The listing builds one solid part. Answer for the finished solid, in the listing's coordinates (mm). Face numbers are marked on the shaded views. A direction names the side the tool comes from. Coordinates: 2 decimals unless noted, no trailing zeros. Order: outer loops, then holes, each group sorted by start corner. A loop starts at its lowest first (then second) coordinate and runs counter-clockwise, first axis right, second up. Notation, with made-up numbers: (6, 40.25) - (36, 40.25) arc R18 ccw to (36, 47.25) - close; hole circle Ø6 at (48.25, 89). An arc over 180 degrees is marked (long way). Use a Markdown table: item, result. Add a question column.
Item 1: The part is cut by section C-C, the plane y = -17. Give the vertices of the cut face in (x, z).
Item 2: The part is cut by section B-B, the plane z = 0. Give the vertices of the cut face in (x, y).
Item 3: For the marked faces 4, 5, 6 and 7, determine the directions among +Z, -Z, +X, -X, +Y, -Y from which every point of the face is accessible in a straight line to the end or side of a thin tool.
Item 4: The part is cut by section D-D, the plane z = 48. Give the vertices of the cut face in (x, y), then the cut area to 3 significant figures.
Item 5: The part is cut by section A-A, the plane x = 0. Give the vertices of the cut face in (y, z).
Item 6: Find the intervals of material crossed by line 1 along Z through (x, y) = (0, -13); line 2 along Z through (x, y) = (5, -23.25); line 3 along X through (y, z) = (-10.25, -48), in increasing order.
Item 7: The mould has two halves that part along X. Classify the marked faces 1, 2 and 3: released by +X, released by -X, zero draft, split by the parting line, or undercut.
Item 8: Flat-ended cylindrical pins translate along their axes: P1, Ø4, axis at y = -14, z = 22.5, coming from the -X side; P2, Ø5.5, axis at y = -6.5, z = 55.5, coming from the -X side; P3, Ø15, axis at x = -50, y = -12, coming from the +Z side; P4, Ø23, axis at x = 0, z = 0, coming from the -Y side. Find the tip coordinate at first contact, or state that the pin passes through.
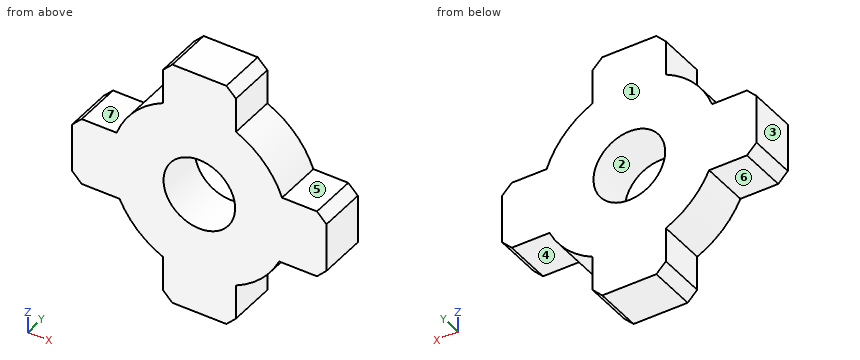
from build123d import *

# Parameters (mm, degrees)
F1_DEPTH = 25.4
F3_D     = 38.1
F4_SIZE  = 5.08
F5_SIZE  = 5.08
F6_SIZE  = 5.08
F7_SIZE  = 5.08
F8_SIZE  = 5.08
F9_SIZE  = 5.08
F10_SIZE = 5.08
F11_SIZE = 5.08


with BuildPart() as f1:
    # F0 (on Front) → F1 (new body)
    with BuildSketch(Plane.XZ):
        with BuildLine():
            Line((-67.625843, -19.898139), (-42.411047, -19.898139))
            ThreePointArc((-42.411047, -19.898139), (-32.947346, -33.303232), (-19.441356, -42.622372))
            Line((-19.441356, -42.622372), (-19.441356, -66.095218))
            Line((-19.441356, -66.095218), (19.480696, -66.095218))
            Line((19.480696, -66.095218), (19.480696, -42.604406))
            ThreePointArc((19.480696, -42.604406), (32.962715, -33.28802), (42.411047, -19.898139))
            Line((42.411047, -19.898139), (67.625843, -19.898139))
            Line((67.625843, -19.898139), (67.625843, 16.122991))
            Line((67.625843, 16.122991), (43.985021, 16.122991))
            ThreePointArc((43.985021, 16.122991), (34.384453, 31.817326), (19.480696, 42.604406))
            Line((19.480696, 42.604406), (19.480696, 66.095218))
            Line((19.480696, 66.095218), (-19.441356, 66.095218))
            Line((-19.441356, 66.095218), (-19.441356, 42.622372))
            ThreePointArc((-19.441356, 42.622372), (-34.369763, 31.833195), (-43.985021, 16.122991))
            Line((-43.985021, 16.122991), (-67.625843, 16.122991))
            Line((-67.625843, 16.122991), (-67.625843, -19.898139))
        make_face()
    extrude(amount=F1_DEPTH)

    # F3 (through all)
    with Locations(Plane(origin=(0, 0, 0), x_dir=(1, 0, 0), z_dir=(0, 1, 0))):
        with Locations((0, 0)):
            Hole(F3_D / 2)

    # F4
    f4_edges = [f1.edges().sort_by_distance(p)[0] for p in [
        (19.480696, -12.7, 66.095218),
    ]]
    chamfer(f4_edges, length=F4_SIZE)

    # F5
    f5_edges = [f1.edges().sort_by_distance(p)[0] for p in [
        (-19.441356, -12.7, 66.095218),
    ]]
    chamfer(f5_edges, length=F5_SIZE)

    # F6
    f6_edges = [f1.edges().sort_by_distance(p)[0] for p in [
        (-67.625843, -12.7, 16.122991),
    ]]
    chamfer(f6_edges, length=F6_SIZE)

    # F7
    f7_edges = [f1.edges().sort_by_distance(p)[0] for p in [
        (-67.625843, -12.7, -19.898139),
    ]]
    chamfer(f7_edges, length=F7_SIZE)

    # F8
    f8_edges = [f1.edges().sort_by_distance(p)[0] for p in [
        (19.480696, -12.7, -66.095218),
    ]]
    chamfer(f8_edges, length=F8_SIZE)

    # F9
    f9_edges = [f1.edges().sort_by_distance(p)[0] for p in [
        (-19.441356, -12.7, -66.095218),
    ]]
    chamfer(f9_edges, length=F9_SIZE)

    # F10
    f10_edges = [f1.edges().sort_by_distance(p)[0] for p in [
        (67.625843, -12.7, 16.122991),
    ]]
    chamfer(f10_edges, length=F10_SIZE)

    # F11
    f11_edges = [f1.edges().sort_by_distance(p)[0] for p in [
        (67.625843, -12.7, -19.898139),
    ]]
    chamfer(f11_edges, length=F11_SIZE)


solid = f1.part
Solution:
| question | item | result |
|---|---|---|
| 1 | outline | (-67.63, -14.82) - (-62.55, -19.9) - (-42.41, -19.9) arc R46.85 ccw to (-19.44, -42.62) - (-19.44, -61.02) - (-14.36, -66.1) - (14.4, -66.1) - (19.48, -61.02) - (19.48, -42.6) arc R46.85 ccw to (42.41, -19.9) - (62.55, -19.9) - (67.63, -14.82) - (67.63, 11.04) - (62.55, 16.12) - (43.99, 16.12) arc R46.85 ccw to (19.48, 42.6) - (19.48, 61.02) - (14.4, 66.1) - (-14.36, 66.1) - (-19.44, 61.02) - (-19.44, 42.62) arc R46.85 ccw to (-43.99, 16.12) - (-62.55, 16.12) - (-67.63, 11.04) - close; hole circle Ø38.1 at (0, 0) |
| 2 | outline | (-67.63, -25.4) - (-19.05, -25.4) - (-19.05, 0) - (-67.63, 0) - close; (19.05, -25.4) - (67.63, -25.4) - (67.63, 0) - (19.05, 0) - close |
| 3 | face 4 | -Z, +X, +Y, -Y |
| 3 | face 5 | +Z, +X, +Y, -Y |
| 3 | face 6 | -Z, -X, +Y, -Y |
| 3 | face 7 | +Z, -X, +Y, -Y |
| 4 | outline | (-19.44, -25.4) - (19.48, -25.4) - (19.48, 0) - (-19.44, 0) - close |
| 4 | area | 989 mm2 |
| 5 | outline | (-25.4, -66.1) - (0, -66.1) - (0, -19.05) - (-25.4, -19.05) - close; (-25.4, 19.05) - (0, 19.05) - (0, 66.1) - (-25.4, 66.1) - close |
| 6 | line 1 | z = -66.1 to -19.05, 19.05 to 66.1 |
| 6 | line 2 | z = -66.1 to -18.38, 18.38 to 66.1 |
| 6 | line 3 | x = -19.44 to 19.48 |
| 7 | face 1 | zero draft |
| 7 | face 2 | undercut |
| 7 | face 3 | released by -X |
| 8 | P1 | stops at x = -42.12 |
| 8 | P2 | stops at x = -19.44 |
| 8 | P3 | stops at z = 19.71 |
| 8 | P4 | passes through |
